Source: CAD feature listing. Evaluate the final solid. Frame: model axes, mm. Face numbers are marked on the shaded views. Round coordinates to 2 decimals unless told otherwise and drop trailing zeros. Loops run counter-clockwise (first coordinate to the right, second up) from the corner with the lowest first, then second, coordinate; pieces in that order, holes last. Notation, with made-up numbers: M 75.25,-22.5 L 99.25,-22.5 A12 ccw 99.25,-2.5 Z; hole C 55.5,35.5 d7. An arc over 180 degrees is marked long. One line per item, written item: value.
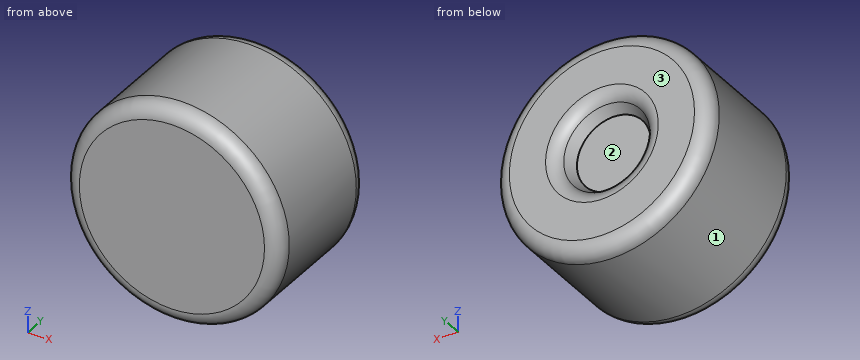
from build123d import *

# Parameters (mm, degrees)
SKETCH1_R           = 284
BOSS_EXTRUDE1_DEPTH = 180
SKETCH2_R           = 125
CUT_EXTRUDE1_DEPTH  = 50
CUT_EXTRUDE1_TAPER  = 29
FILLET1_R           = 40
FILLET2_R           = 40
FILLET3_R           = 40


with BuildPart() as part:
    # Sketch1 → Boss-Extrude1 (new body, symmetric)
    with BuildSketch(Plane(origin=(0, 0, 0), x_dir=(1, 0, 0), z_dir=(0, 1, 0))):
        Circle(SKETCH1_R)
    extrude(amount=BOSS_EXTRUDE1_DEPTH, both=True)

    # Sketch2 → Cut-Extrude1 (cut)
    with BuildSketch(Plane(origin=(0, 180, 0), x_dir=(1, 0, 0), z_dir=(0, 1, 0))):
        Circle(SKETCH2_R)
    extrude(amount=-CUT_EXTRUDE1_DEPTH, taper=CUT_EXTRUDE1_TAPER, mode=Mode.SUBTRACT)

    # Fillet1
    fillet1_edges = [part.edges().sort_by_distance(p)[0] for p in [
        (-284, 180, 0),
    ]]
    fillet(fillet1_edges, radius=FILLET1_R)

    # Fillet2
    fillet2_edges = [part.edges().sort_by_distance(p)[0] for p in [
        (-125, 180, 0),
    ]]
    fillet(fillet2_edges, radius=FILLET2_R)

    # Fillet3
    fillet3_edges = [part.edges().sort_by_distance(p)[0] for p in [
        (-284, -180, 0),
    ]]
    fillet(fillet3_edges, radius=FILLET3_R)


solid = part.part
1. Pin query (flat end, axial travel): pin 1 (3 mm diameter, centred on x = -77.5, y = -77.5, fed in from -Z); pin 2 (4 mm diameter, centred on y = -25.5, z = 196.5, fed in from +X); pin 3 (1 mm diameter, centred on x = -22, z = 79, fed in from +Y). Return the tip coordinate at first contact, or that it passes through.
Report:
pin 1: stops at z = -273.64
pin 2: stops at x = 206.94
pin 3: stops at y = 130
2. Section query B-B (y = -86.5). Return the cut outline in (x, z).
Report:
outline: C 0,0 d568
3. Ray query, line 1 (Y direction, x = 12, z = -92); line 2 (Y direction, x = -16, z = 145); line 3 (X direction, y = -43, z = -180). Return the intervals inside material, ascending. Write a range as [from, to].
Report:
line 1: y = [-180, 130]
line 2: y = [-180, 179.91]
line 3: x = [-219.67, 219.67]
4. Section query A-A (x = 0). Return the cut outline in (y, z), and give its area (3 significant figures).
Report:
outline: M -180,-244 A40 ccw -140,-284 L 140,-284 A40 ccw 180,-244 L 180,-148.56 A40 ccw 159.39,-113.58 L 130,-97.28 L 130,97.28 L 159.39,113.58 A40 ccw 180,148.56 L 180,244 A40 ccw 140,284 L -140,284 A40 ccw -180,244 Z
area: 192,000 mm2
5. Pull-direction query (X, two-part tool) for the marked faces 1, 2 and 3; classes: released by +X, released by -X, zero draft, split by the parting line, or undercut.
Report:
face 1: split by the parting line
face 2: undercut
face 3: zero draft
